For this review, use the dimensioned drawing (mm, ordinates from the lowest corner) and the shaded views. A direction names the side the tool comes from. Give positions to 0.01 mm unless a question says otherwise; leave off trailing zeros. Order: outer loops, then holes, each group sorted by start corner. A loop starts at its lowest first (then second) coordinate and runs counter-clockwise, first axis right, second up. Notation, with made-up numbers: (-4, 80) -> (11, 80) arc R23 cw to (11, 92) -> close; hole circle Ø1 at (12, 65.5). An arc over 180 degrees is marked (long way). Answer as a JSON object with one key per item and string values. Group by question number.
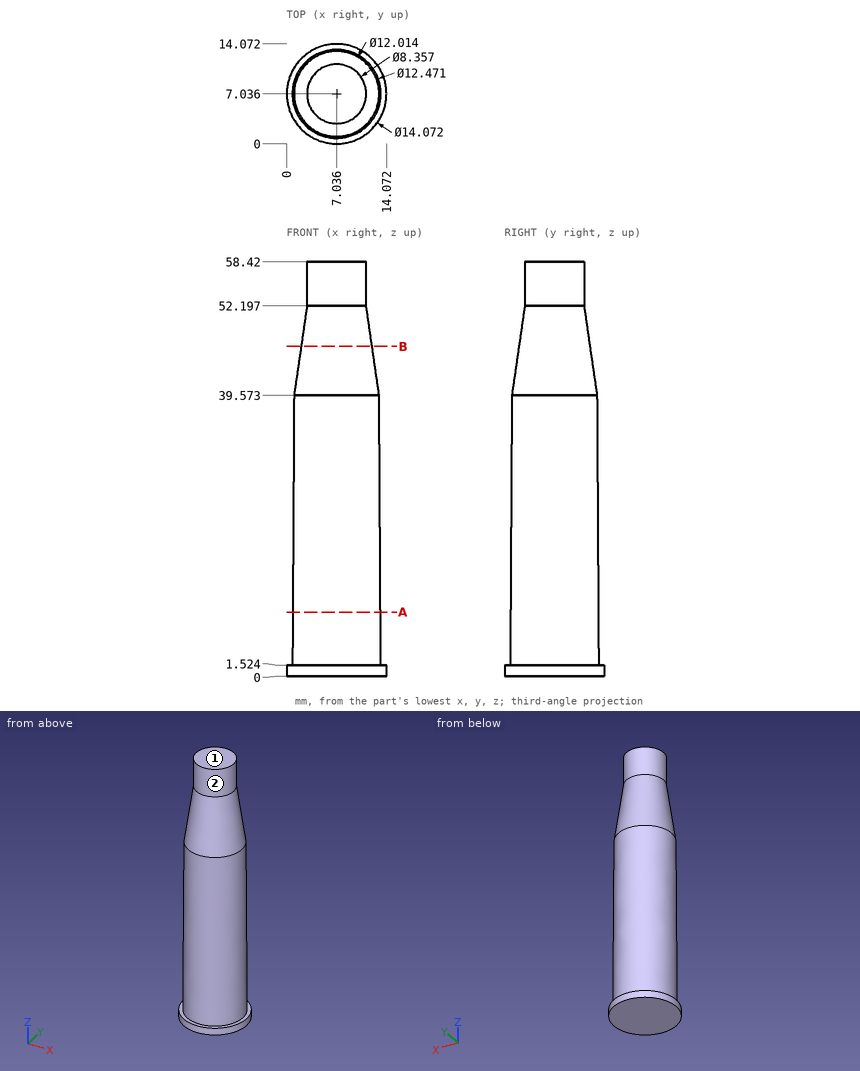
1. For probe 1 along Z at (x, y) = (1.5, 10.75); probe 2 along X at (y, z) = (6.75, 17.5); probe 3 along X at (y, z) = (11.5, 45.5), list the stretches that pass through material, from the lowest coordinate up. Write a range as [from, to].
2. For pin 1 (2 mm diameter, centred on x = 11.5, z = 22, fed in from +Y); pin 2 (4 mm diameter, centred on y = 7.5, z = 42.5, fed in from -X); pin 3 (8 mm diameter, centred on x = 11, z = 28.5, fed in from +Y) (1 decimal); pin 4 (5 mm diameter, centred on x = 9.5, y = 3.5, fed in from +Z), all flat-tipped, find the tip position at first contact; note any pin that passes through.
3. Take a section at A-A on z = 9. Give the boundary of the cut face in (x, y) (1 decimal), plus the area to 3 significant figures.
4. Machinability: for the marked faces 1 and 2, which of the approach directions +Z, -Z, +X, -X, +Y, -Y give a long, thin tool a straight path to every point of the face, cutting with its end or side? Answer none if there is none.
5. Take a section at B-B on z = 46.5. Give the boundary of the cut face in (x, y) (1 decimal).
Checks:
{
 "1": {"probe 1": "z = [0, 1.52]", "probe 2": "x = [0.9, 13.17]", "probe 3": "x = [4.47, 9.6]"},
 "2": {"pin 1": "stops at y = 12.07", "pin 2": "stops at x = 1.17", "pin 3": "stops at y = 13.1", "pin 4": "stops at z = 58.42"},
 "3": {"outline": "circle Ø12.4 at (7, 7)", "area": "120 mm2"},
 "4": {"face 1": "+Z, +X, -X, +Y, -Y", "face 2": "+Z"},
 "5": {"outline": "circle Ø10 at (7, 7)"}
}
